For this review, take the finished solid that the model builds, in its own axes (mm). Coordinates: 2 decimals unless noted, no trailing zeros. Loops run counter-clockwise (first coordinate to the right, second up) from the corner with the lowest first, then second, coordinate; pieces in that order, holes last. Notation, with made-up numbers: M -9,75 L 3,75 A32 ccw 3,107 Z; hole C -25,22.5 d9. An arc over 180 degrees is marked long. Use one line per item in the form item = value.
Solid Edge part; units mm, degrees
sketch "Sketch1" plane through (0, 0, 0) normal (0, -1, 0) x (1, 0, 0)
  circle A0 centre (0, 0) radius 11
  circle A1 centre (0, 0) radius 9
extrude "Protrusion1" add sketch "Sketch1" against normal blind 7
sketch "Sketch2" plane through (0, 0, 0) normal (0, 0, 1) x (1, 0, 0)
  circle A0 centre (-7.25, 3.5) radius 2
revolve "RevolvedCutout1" cut sketch "Sketch2" angle 360 about axis through (0, 0, 0) along (0, 1, 0)
chamfer "Chanfrein_1" distance 0.5 angle 45 2 edges at (-11, 0, 0) (-11, 7, 0)
chamfer "Chanfrein_2" distance 0.25 angle 45 2 edges at (-9, 0, 0) (-9, 7, 0)
properties material "Steel"
1. Draft analysis for pull direction X (two halves, no side actions). For faces 1 (the face through (-2.38, 3.46, -10.74)), 2 (the face through (-1.172, 5.593, 8.923)), 3 (the face through (-9, 0, -4)), state which applies: +X half, -X half, draft (parallel to the pull), parting line (faces both ways), or undercut.
Computed values:
face_1 = parting line
face_2 = undercut
face_3 = draft
2. Consider section C-C on y = 6. Write out the cut boundary in (x, z).
Computed values:
outline = C 0,0 d22; hole C 0,0 d18
3. For pin 1 Ø2 at (x, z) = (-4, 6.5) entering from +Y; pin 2 Ø1 at (x, y) = (2, 3.5) entering from -Z; pin 3 Ø3 at (x, y) = (-6.5, 3.5) entering from +Z, all flat-tipped, find the tip position at first contact; note any pin that passes through.
Computed values:
pin_1 = through
pin_2 = -10.9
pin_3 = 9.8
4. Wall thickness on line 1 along Z through (x, y) = (0, 1.4); line 2 along X through (y, z) = (1.75, -0.75); line 3 along X through (y, z) = (4, 1.5): over which ranges is each line inside the solid? List them lowest first. Write a range as from..to.
Computed values:
line_1 = -11..-9, 9..11
line_2 = -10.97..-8.97, 8.97..10.97
line_3 = -10.9..-9.06, 9.06..10.9
5. Consider section A-A on z = 0. Write out the cut boundary in (x, y), plus the area to 3 significant figures.
Computed values:
outline = M -11,0.5 L -10.5,0 L -9.25,0 L -9,0.25 L -9,2.53 A2 cw -9,4.47 L -9,6.75 L -9.25,7 L -10.5,7 L -11,6.5 Z; M 9,0.25 L 9.25,0 L 10.5,0 L 11,0.5 L 11,6.5 L 10.5,7 L 9.25,7 L 9,6.75 L 9,4.47 A2 cw 9,2.53 Z
area = 26.7 mm2
6. Consider section B-B on x = 0. Write out the cut boundary in (y, z).
Computed values:
outline = M 0,-10.5 L 0.5,-11 L 6.5,-11 L 7,-10.5 L 7,-9.25 L 6.75,-9 L 4.47,-9 A2 cw 2.53,-9 L 0.25,-9 L 0,-9.25 Z; M 0,9.25 L 0.25,9 L 2.53,9 A2 cw 4.47,9 L 6.75,9 L 7,9.25 L 7,10.5 L 6.5,11 L 0.5,11 L 0,10.5 Z
